Geometry check sheet. Reference: the model listing, model coordinates, mm. A direction names the side the tool comes from. Give positions to 0.01 mm unless a question says otherwise; leave off trailing zeros. Order: outer loops, then holes, each group sorted by start corner. A loop starts at its lowest first (then second) coordinate and runs counter-clockwise, first axis right, second up.
```python
from build123d import *

# Parameters (mm, degrees)
BOSS_EXTRUDE1_DEPTH      = 88.9
CUT_EXTRUDE2_DEPTH       = 241.232341963
CUT_EXTRUDE2_DEPTH_BACK  = 241.232341963
SKETCH3_R                = 28.575
CUT_EXTRUDE5_DEPTH       = 28.575
CUT_EXTRUDE6_DEPTH       = 243.134084755
CUT_EXTRUDE6_DEPTH_BACK  = 243.134084755
SKETCH4_R                = 12.7
CUT_EXTRUDE7_DEPTH       = 261.369359036
CUT_EXTRUDE7_DEPTH_BACK  = 261.369359036
CUT_EXTRUDE8_DEPTH       = 261.369359036
CUT_EXTRUDE8_DEPTH_BACK  = 12.7
SKETCH6_R                = 6.35
SKETCH7_R                = 6.35
CUT_EXTRUDE9_DEPTH       = 12.7
SKETCH12_R               = 12.7
CUT_EXTRUDE13_DEPTH      = 3.175
CUT_EXTRUDE14_DEPTH      = 158.75
CUT_EXTRUDE14_DEPTH_BACK = 253.187753717
CUT_EXTRUDE14_START      = -12.7
SKETCH14_R               = 1.5875
CUT_EXTRUDE15_DEPTH      = 261.369359036
CUT_EXTRUDE15_DEPTH_BACK = 261.369359036
SKETCH15_W               = 158.75
SKETCH15_H               = 174.625
SKETCH17_R               = 6.35
BOSS_EXTRUDE3_DEPTH      = 9.525
CHAMFER2_SIZE            = 1.5875
CUT_EXTRUDE16_DEPTH      = 198.208141947
CUT_EXTRUDE16_DEPTH_BACK = 5.5626
SKETCH18_R               = 11.1125


with BuildPart() as part:
    # Sketch1 → Boss-Extrude1 (new body)
    with BuildSketch(Plane.XY):
        Polygon((0, 0), (0, -174.625), (171.45, -174.625), (171.45, 0), (158.75, 0), (158.75, -142.875), (12.7, -142.875), (12.7, 0), align=None)
    extrude(amount=BOSS_EXTRUDE1_DEPTH)

    # Sketch2 → Cut-Extrude2 (cut, two sides: drawn at the far end of the back side and taken through both)
    with BuildSketch(Plane(origin=(0, -142.875, 0), x_dir=(1, 0, 0), z_dir=(0, 1, 0)).offset(-CUT_EXTRUDE2_DEPTH_BACK)):
        Polygon((158.75, 0), (12.7, 0), (12.7, -25.4), (85.724999876, -25.4), (158.75, -25.4), align=None)
    extrude(amount=CUT_EXTRUDE2_DEPTH + CUT_EXTRUDE2_DEPTH_BACK, mode=Mode.SUBTRACT)

    # Sketch3 → Cut-Extrude5 (cut)
    with BuildSketch(Plane.XZ.offset(174.625)):
        with Locations((85.725, 57.15)):
            Circle(SKETCH3_R)
    extrude(amount=-CUT_EXTRUDE5_DEPTH, mode=Mode.SUBTRACT)

    # Sketch4 → Cut-Extrude6 (cut, two sides: drawn at the far end of the back side and taken through both)
    with BuildSketch(Plane.XZ.offset(146.05).offset(-CUT_EXTRUDE6_DEPTH_BACK)):
        with Locations((85.725, 57.15)):
            Circle(SKETCH4_R)
    extrude(amount=CUT_EXTRUDE6_DEPTH + CUT_EXTRUDE6_DEPTH_BACK, mode=Mode.SUBTRACT)

    # Sketch5 → Cut-Extrude7 (cut, two sides: drawn at the far end of the back side and taken through both)
    with BuildSketch(Plane(origin=(171.45, 0, 0), x_dir=(0, 0, -1), z_dir=(1, 0, 0)).offset(-CUT_EXTRUDE7_DEPTH_BACK)):
        with BuildLine():
            Line((0, -174.625), (0, -114.3))
            ThreePointArc((0, -114.3), (-0.597344099, -119.776153781), (-2.361280333, -124.994736842))
            Line((-2.361280333, -124.994736842), (-25.4, -174.625))
            Line((-25.4, -174.625), (0, -174.625))
        make_face()
        with BuildLine():
            Line((-39.269490456, -98.025866748), (-71.745289975, -22.119448379))
            ThreePointArc((-71.745289975, -22.119448379), (-70.400400796, -7.131859618), (-57.149999966, 0))
            Line((-57.149999966, 0), (-88.9, 0))
            Line((-88.9, 0), (-88.9, -142.875))
            Line((-88.9, -142.875), (-50.8, -142.875))
            Line((-50.8, -142.875), (-39.583234749, -118.711720996))
            ThreePointArc((-39.583234749, -118.711720996), (-37.224875429, -108.402184034), (-39.269490456, -98.025866748))
        make_face()
        with BuildLine():
            Line((0, 0), (-57.149999966, 0))
            ThreePointArc((-57.149999966, 0), (-48.406859618, -2.624599204), (-42.554710025, -9.630551621))
            Line((-42.554710025, -9.630551621), (-2.047536041, -104.308882594))
            ThreePointArc((-2.047536041, -104.308882594), (-0.51714863, -109.200616928), (0, -114.3))
            Line((0, -114.3), (0, 0))
        make_face()
    extrude(amount=CUT_EXTRUDE7_DEPTH + CUT_EXTRUDE7_DEPTH_BACK, mode=Mode.SUBTRACT)

    # Sketch6 → Cut-Extrude8 (cut, two sides: drawn at the far end of the back side and taken through both)
    with BuildSketch(Plane(origin=(171.45, 0, 0), x_dir=(0, 0, -1), z_dir=(1, 0, 0)).offset(-CUT_EXTRUDE8_DEPTH_BACK)):
        with Locations(Location((-57.15, -15.875, 0), (0, 0, 90))):
            Circle(SKETCH6_R)
    extrude(amount=CUT_EXTRUDE8_DEPTH + CUT_EXTRUDE8_DEPTH_BACK, mode=Mode.SUBTRACT)

    # Sketch7 → Cut-Extrude9 (cut)
    with BuildSketch(Plane(origin=(12.7, 0, 0), x_dir=(0, 0, -1), z_dir=(1, 0, 0))):
        with Locations(Location((-57.15, -15.875, 0), (0, 0, 90))):
            Circle(SKETCH7_R)
    extrude(amount=-CUT_EXTRUDE9_DEPTH, mode=Mode.SUBTRACT)

    # Sketch12 → Cut-Extrude13 (cut)
    with BuildSketch(Plane(origin=(12.7, 0, 0), x_dir=(0, 0, -1), z_dir=(1, 0, 0))):
        with Locations((-57.15, -15.875)):
            Circle(SKETCH12_R)
    extrude(amount=-CUT_EXTRUDE13_DEPTH, mode=Mode.SUBTRACT)

    # Sketch14 → Cut-Extrude14 (cut, two sides: drawn at the far end of the back side and taken through both)
    with BuildSketch(Plane(origin=(12.7, 0, 0), x_dir=(0, 0, -1), z_dir=(1, 0, 0)).offset(CUT_EXTRUDE14_START - CUT_EXTRUDE14_DEPTH_BACK)):
        with Locations(Location((-53.770765225, -24.780413934, 0), (0, 0, 90))):
            Circle(SKETCH14_R)
        with Locations(Location((-66.551932086, -14.348796194, 0), (0, 0, 90))):
            Circle(SKETCH14_R)
        with Locations(Location((-51.12730269, -8.495789872, 0), (0, 0, 90))):
            Circle(SKETCH14_R)
    extrude(amount=CUT_EXTRUDE14_DEPTH + CUT_EXTRUDE14_DEPTH_BACK, mode=Mode.SUBTRACT)

    # Sketch15 → Cut-Extrude15 (cut, two sides: drawn at the far end of the back side and taken through both)
    with BuildSketch(Plane.XY.offset(88.9).offset(-CUT_EXTRUDE15_DEPTH_BACK)):
        with Locations((79.375, -87.3125)):
            Rectangle(SKETCH15_W, SKETCH15_H)
    extrude(amount=CUT_EXTRUDE15_DEPTH + CUT_EXTRUDE15_DEPTH_BACK, mode=Mode.SUBTRACT)

    # Sketch17 → Boss-Extrude3 (add)
    with BuildSketch(Plane.ZY.offset(-158.75)):
        with Locations(Location((76.2, -158.75, 0), (0, 0, 90))):
            Circle(SKETCH17_R)
        with Locations(Location((38.1, -158.75, 0), (0, 0, 90))):
            Circle(SKETCH17_R)
    extrude(amount=BOSS_EXTRUDE3_DEPTH)

    # Chamfer2
    chamfer2_edges = [part.edges().sort_by_distance(p)[0] for p in [
        (149.225, -165.1, 76.2),
        (149.225, -165.1, 38.1),
    ]]
    chamfer(chamfer2_edges, length=CHAMFER2_SIZE)

    # Sketch18 → Cut-Extrude16 (cut, two sides: drawn at the far end of the back side and taken through both)
    with BuildSketch(Plane(origin=(171.45, 0, 0), x_dir=(0, 0, -1), z_dir=(1, 0, 0)).offset(-CUT_EXTRUDE16_DEPTH_BACK)):
        with Locations(Location((-57.15, -15.875, 0), (0, 0, 270))):
            Circle(SKETCH18_R)
    extrude(amount=CUT_EXTRUDE16_DEPTH + CUT_EXTRUDE16_DEPTH_BACK, mode=Mode.SUBTRACT)


solid = part.part
```
Q1. Gauge pin test, flat ends, axial feed: P1, Ø2, axis at x = 161, y = -43, coming from the -Z side; P2, Ø1, axis at x = 158.5, y = -79, coming from the +Z side; P3, Ø1.5, axis at x = 154.5, z = 71, coming from the +Y side. Record the tip position at first contact, or that the pin passes through.
Q2. Thickness scan on L1, parallel to Y at x = 169.6, z = 57.15 (1 decimal); L2, parallel to Y at x = 162, z = 57.15 (3 decimals); L3, parallel to X at y = -153.5, z = 23.5. Record the ranges inside material, lowest first.
Q3. Release check for a two-part mould opening along Z. For faces 5 (the face through (165, -142.875, 70)), 6 (the face through (154.837, -152.693, 36.193)), 7 (the face through (165.01, -130.96, 45.27)) record: pulls with the +Z half, pulls with the -Z half, needs draft (parallel to the pull), parting line crosses it, or undercut.
Q4. Cross-section at D-D, the plane z = 13. Record the boundary of the cut face in (x, y), and give its area (3 significant figures).
Q5. Access from +Z, -Z, +X, -X, +Y, -Y to the whole of each face (thin tool, end or side, straight path). Record for faces 1 (the face through (165.887, -21, 62)), 2 (the face through (154.837, -152.693, 74.293)), 3 (the face through (165.01, -60.6, 55.28)), 4 (the face through (149.225, -159, 76)).
Answers follow:
1. P1: stops at z = 27.85
1. P2: stops at z = 47.59
1. P3: stops at y = -154.22
2. L1: y = -174.6 to -142.9, -56.2 to -27, -4.8 to 0
2. L2: y = -174.625 to -142.875, -56.233 to -22.225, -9.525 to 0
2. L3: x = 158.75 to 171.45
3. face 5: needs draft
3. face 6: undercut
3. face 7: pulls with the +Z half
4. outline: (158.75, -147.91) - (171.45, -147.91) - (171.45, -78.71) - (158.75, -78.71) - close
4. area: 879 mm2
5. face 1: +X
5. face 2: -X
5. face 3: +Z, +X, -X
5. face 4: +Z, -Z, -X, +Y, -Y
